Autodesk Inventor part; units mm, degrees
ref_plane "YZ Plane" through (0, 0, 0) normal (1, 0, 0) x (0, 1, 0)
ref_plane "XZ Plane" through (0, 0, 0) normal (0, 1, 0) x (-1, 0, 0)
ref_plane "XY Plane" through (0, 0, 0) normal (0, 0, 1) x (1, 0, 0)
sketch "Эскиз1" plane through (0, 0, 0) normal (0, 0, 1) x (1, 0, 0)
  circle A0 centre (0, 0) radius 40
  circle A1 centre (0, 0) radius 30 construction
  line L0 (17.5791, -24.31) -> (-17.6879, -24.2309) construction
  line L1 (-17.6879, -24.2309) -> (-28.5108, 9.3345) construction
  line L2 (-28.5108, 9.3345) -> (0.0673, 29.9999) construction
  line L3 (0.0673, 29.9999) -> (28.5524, 9.2065) construction
  line L4 (28.5524, 9.2065) -> (17.5791, -24.31) construction
  circle A2 centre (-28.5108, 9.3345) radius 5
  circle A3 centre (0.0673, 29.9999) radius 5
  circle A4 centre (28.5524, 9.2065) radius 5
  circle A5 centre (17.5791, -24.31) radius 5
  circle A6 centre (-17.6879, -24.2309) radius 5
  circle A7 centre (0, 0) radius 60 construction
  line L5 (0, 0) -> (42.4264, 42.4264)
  line L6 (0, 0) -> (60, 0) construction
  line L7 (42.4264, 42.4264) -> (-42.4264, 42.4264) construction
  line L8 (-42.4264, 42.4264) -> (-42.4264, -42.4264) construction
  line L9 (42.4264, -42.4264) -> (42.4264, 42.4264) construction
  line L10 (-42.4264, -42.4264) -> (42.4264, -42.4264) construction
  arc A8 (42.4264, 42.4264) -> (-42.4264, 42.4264) centre (0, 0) ccw construction
  arc A9 (49.4975, 49.4975) -> (-49.4975, 49.4975) centre (0, 0) ccw
  arc A10 (35.3553, 35.3553) -> (-35.3553, 35.3553) centre (0, 0) ccw
  arc A11 (35.3553, 35.3553) -> (49.4975, 49.4975) centre (42.4264, 42.4264) ccw
  arc A12 (-49.4975, 49.4975) -> (-35.3553, 35.3553) centre (-42.4264, 42.4264) ccw
  arc A13 (42.4264, 42.4264) -> (-42.4264, 42.4264) centre (0, 0) ccw construction
  arc A14 (53.033, 53.033) -> (-53.033, 53.033) centre (0, 0) ccw
  arc A15 (-42.4264, -42.4264) -> (42.4264, -42.4264) centre (0, 0) ccw construction
  arc A16 (-49.4975, -49.4975) -> (49.4975, -49.4975) centre (0, 0) ccw
  arc A17 (-35.3553, -35.3553) -> (35.3553, -35.3553) centre (0, 0) ccw
  arc A18 (-35.3553, -35.3553) -> (-49.4975, -49.4975) centre (-42.4264, -42.4264) ccw
  arc A19 (49.4975, -49.4975) -> (35.3553, -35.3553) centre (42.4264, -42.4264) ccw
  arc A20 (-42.4264, -42.4264) -> (42.4264, -42.4264) centre (0, 0) ccw construction
  arc A21 (-54.4472, -54.4472) -> (54.4472, -54.4472) centre (0, 0) ccw
  arc A22 (-33.9116, 21.2132) -> (-39.6003, 27.695) centre (-38.6583, 22.7846) ccw
  arc A23 (39.6003, 27.695) -> (33.9116, 21.2132) centre (38.6583, 22.7846) ccw
  arc A24 (-38.6583, -25.8493) -> (-33.9116, -21.2132) centre (-38.8988, -20.8551) ccw
  arc A25 (33.9116, -21.2132) -> (38.6583, -25.8493) centre (38.8988, -20.8551) ccw
  arc A26 (-53.033, 53.033) -> (-39.6003, 27.695) centre (-42.4264, 42.4264) ccw
  arc A27 (39.6003, 27.695) -> (53.033, 53.033) centre (42.4264, 42.4264) ccw
  arc A28 (-38.6583, -25.8493) -> (-54.4472, -54.4472) centre (-42.4264, -42.4264) ccw
  arc A29 (54.4472, -54.4472) -> (38.6583, -25.8493) centre (42.4264, -42.4264) ccw
  dimension "d1" = 60
  dimension "d0" = 80
  dimension "d8" = 10
  dimension "d9" = 33.5165
  dimension "d22" = 120
  dimension "d23" = 60
  dimension "d24" = 45
  dimension "d25" = 20
  dimension "d27" = 20
  dimension "d29" = 5
  dimension "d31" = 5
  dimension "d32" = 5
  dimension "d33" = 5
  dimension "d34" = 2.8261
  dimension "d35" = 3.5276
  dimension "d36" = 20.8551
  dimension "d37" = 76.338
  dimension "d38" = 76.3381
  dimension "d39" = 81.0847
  dimension "d40" = 15
  dimension "d41" = 17
sketch "Эскиз2" plane through (0, 0, 0) normal (0, 0, 1) x (1, 0, 0)
  point P0 (0, 0)
extrude "Выдавливание1" add sketch "Эскиз1" along normal blind 10
properties part number "пр3дет1"
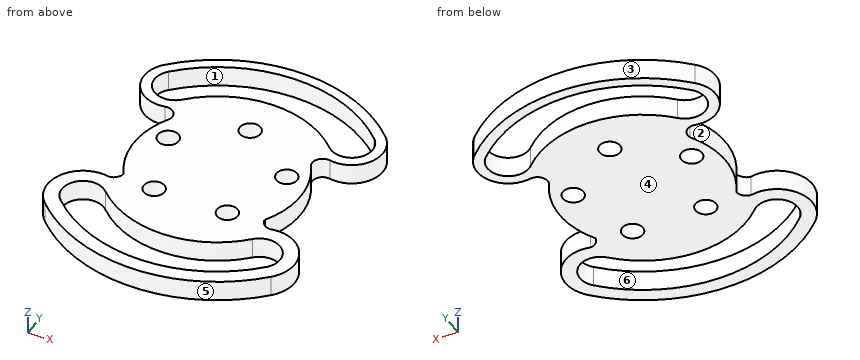
Model file for the job. Use its own axes, mm. Face numbers are marked on the shaded views. A direction names the side the tool comes from. Give positions to 0.01 mm unless a question says otherwise; leave off trailing zeros. Loops run counter-clockwise (first coordinate to the right, second up) from the corner with the lowest first, then second, coordinate; pieces in that order, holes last.
Item 1: Which spindle directions (+Z, -Z, +X, -X, +Y, -Y) get a long thin tool onto all of the face, cutting with end or side? Do the marked faces 1 and 2. Say none if no direction does.
Check values:
face 1: +Z, -Z
face 2: +Z, -Z, -X
Item 2: Slice it at D-D (x = -11). Write the cut outline in (y, z), plus the area to 3 significant figures.
Check values:
outline: (-76.21, 0) - (-69.13, 0) - (-69.13, 10) - (-76.21, 10) - close; (-48.77, 0) - (48.77, 0) - (48.77, 10) - (-48.77, 10) - close; (69.13, 0) - (74.19, 0) - (74.19, 10) - (69.13, 10) - close
area: 1,100 mm2
Item 3: Slice it at A-A (x = 26.5). Write the cut outline in (y, z).
Check values:
outline: (-72.3, 0) - (-64.79, 0) - (-64.79, 10) - (-72.3, 10) - close; (-42.4, 0) - (4.65, 0) - (4.65, 10) - (-42.4, 10) - close; (13.77, 0) - (42.4, 0) - (42.4, 10) - (13.77, 10) - close; (64.79, 0) - (70.16, 0) - (70.16, 10) - (64.79, 10) - close
Item 4: Drill centre lines: line 1 along X through (y, z) = (29.5, 1.75); line 2 along X through (y, z) = (-33.5, 9.25); line 3 along Y through (x, z) = (-3, 3). Where is each one in solid material? Low to high.
Check values:
line 1: x = -50.04 to -4.91, 5.04 to 50.04
line 2: x = -56.89 to -46.93, -37.92 to 37.92, 46.93 to 56.89
line 3: y = -76.94 to -69.94, -49.91 to 26.05, 33.95 to 49.91, 69.94 to 74.94
Item 5: Mould opens along Y. For the marked faces 3, 4, 5 and 6 say: +Y half, -Y half, draft (parallel to the pull), parting line (faces both ways), or undercut.
Check values:
face 3: +Y half
face 4: draft
face 5: -Y half
face 6: undercut
Item 6: Slice it at C-C (y = 55.5). Write the cut outline in (x, z), plus the area to 3 significant figures.
Check values:
outline: (-50.45, 0) - (-42.66, 0) - (-42.66, 10) - (-50.45, 10) - close; (42.66, 0) - (50.45, 0) - (50.45, 10) - (42.66, 10) - close
area: 156 mm2
Item 7: Drop flat-ended pins along their axis: P1, Ø1.5, axis at y = -0.5, z = 6, coming from the -X side; P2, Ø1.5, axis at x = -10.5, z = 7, coming from the +Y side; P3, Ø11.5, axis at x = 17.58, y = -24.31, coming from the +Z side; P4, Ø2, axis at y = 45.5, z = 3, coming from the +X side. Give the stop position or say it passes through.
Check values:
P1: stops at x = -40
P2: stops at y = 74.36
P3: stops at z = 10
P4: stops at x = 57.28
Item 8: Slice it at B-B (z = 6). Write the cut outline in (x, y) (1 decimal), plus the area to 3 significant figures.
Check values:
outline: (-54.4, -54.4) arc R77 ccw to (54.4, -54.4) arc R17 ccw to (38.7, -25.8) arc R5 cw to (33.9, -21.2) arc R40 ccw to (33.9, 21.2) arc R5 cw to (39.6, 27.7) arc R15 ccw to (53, 53) arc R75 ccw to (-53, 53) arc R15 ccw to (-39.6, 27.7) arc R5 cw to (-33.9, 21.2) arc R40 ccw to (-33.9, -21.2) arc R5 cw to (-38.7, -25.8) arc R17 ccw to start; hole (-49.5, -49.5) arc R70 ccw to (49.5, -49.5) arc R10 ccw to (35.4, -35.4) arc R50 cw to (-35.4, -35.4) arc R10 ccw to start; hole (-49.5, 49.5) arc R10 ccw to (-35.4, 35.4) arc R50 cw to (35.4, 35.4) arc R10 ccw to (49.5, 49.5) arc R70 ccw to start; hole circle Ø10 at (-28.5, 9.3); hole circle Ø10 at (-17.7, -24.2); hole circle Ø10 at (0.1, 30); hole circle Ø10 at (17.6, -24.3); hole circle Ø10 at (28.6, 9.2)
area: 8,550 mm2
